For this review, take the finished solid that the model builds, in its own axes (mm). A direction names the side the tool comes from. Give positions to 0.01 mm unless a question says otherwise; leave off trailing zeros. Loops run counter-clockwise (first coordinate to the right, second up) from the corner with the lowest first, then second, coordinate; pieces in that order, holes last. Notation, with made-up numbers: (51.25, 9.25) - (73.25, 9.25) arc R15 ccw to (73.25, 37.25) - close; hole circle Ø11 at (48.25, 88). An arc over 180 degrees is marked (long way). Put each result on its own line as item: value. Start each with the question number.
from build123d import *

# Parameters (mm, degrees)
SKICA1_W                 = 55.6
SKICA1_H                 = 55.6
SKICA1_W_2               = 53.6
SKICA1_H_2               = 53.6
P_IDAT_VYSUNUT_M1_DEPTH  = 10
SKICA3_W                 = 5.8
SKICA3_H                 = 5.8
P_IDAT_VYSUNUT_M2_DEPTH  = 10
ZAOBLIT1_R               = 2.5
SKICA4_R                 = 2.4
ODEBRAT_VYSUNUT_M1_DEPTH = 8
SKICA5_R                 = 0.5
ODEBRAT_VYSUNUT_M2_DEPTH = 2
SKICA6_W                 = 48.6
SKICA6_H                 = 48
ODEBRAT_VYSUNUT_M3_DEPTH = 1.5
SKICA7_W                 = 5.5
SKICA7_H                 = 10.4
ODEBRAT_VYSUNUT_M4_DEPTH = 55.6


with BuildPart() as part:
    # Skica1 → Přidat vysunutím1 (new body)
    with BuildSketch(Plane.XY):
        Rectangle(SKICA1_W, SKICA1_H)
        Rectangle(SKICA1_W_2, SKICA1_H_2, mode=Mode.SUBTRACT)
    extrude(amount=P_IDAT_VYSUNUT_M1_DEPTH)

    # Skica3 → Přidat vysunutím2 (add)
    with BuildSketch(Plane(origin=(0, 0, 0), x_dir=(-1, 0, 0), z_dir=(0, 0, -1))):
        with Locations((23.9, -23.9)):
            Rectangle(SKICA3_W, SKICA3_H)
        with Locations((23.9, 23.9)):
            Rectangle(SKICA3_W, SKICA3_H)
        with Locations((-23.9, -23.9)):
            Rectangle(SKICA3_W, SKICA3_H)
        with Locations((-23.9, 23.9)):
            Rectangle(SKICA3_W, SKICA3_H)
    extrude(amount=-P_IDAT_VYSUNUT_M2_DEPTH)

    # Zaoblit1
    zaoblit1_edges = [part.edges().sort_by_distance(p)[0] for p in [
        (-21, 21, 5),
        (-21, -21, 5),
        (21, -21, 5),
        (21, 21, 5),
    ]]
    fillet(zaoblit1_edges, radius=ZAOBLIT1_R)

    # Skica4 → Odebrat vysunutím1 (cut)
    with BuildSketch(Plane(origin=(0, 0, 0), x_dir=(-1, 0, 0), z_dir=(0, 0, -1))):
        with Locations((23.9, 23.9)):
            Circle(SKICA4_R)
        with Locations((23.9, -23.9)):
            Circle(SKICA4_R)
        with Locations((-23.9, -23.9)):
            Circle(SKICA4_R)
        with Locations((-23.9, 23.9)):
            Circle(SKICA4_R)
    extrude(amount=-ODEBRAT_VYSUNUT_M1_DEPTH, mode=Mode.SUBTRACT)

    # Skica5 → Odebrat vysunutím2 (cut)
    with BuildSketch(Plane(origin=(0, 0, 8), x_dir=(-1, 0, 0), z_dir=(0, 0, -1))):
        with Locations((24.868963017, 24.910500208)):
            Circle(SKICA5_R)
        with Locations((-24.910500208, 24.868963017)):
            Circle(SKICA5_R)
        with Locations((24.910500208, -24.868963017)):
            Circle(SKICA5_R)
        with Locations((-24.868963017, -24.910500208)):
            Circle(SKICA5_R)
    extrude(amount=-ODEBRAT_VYSUNUT_M2_DEPTH, mode=Mode.SUBTRACT)

    # Skica6 → Odebrat vysunutím3 (cut)
    with BuildSketch(Plane.XY.offset(10)):
        Rectangle(SKICA6_W, SKICA6_H)
    extrude(amount=-ODEBRAT_VYSUNUT_M3_DEPTH, mode=Mode.SUBTRACT)

    # Skica7 → Odebrat vysunutím4 (cut)
    with BuildSketch(Plane(origin=(27.8, 0, 0), x_dir=(0, 0, -1), z_dir=(1, 0, 0))):
        with Locations((-4.75, 0)):
            Rectangle(SKICA7_W, SKICA7_H)
    extrude(amount=-ODEBRAT_VYSUNUT_M4_DEPTH, mode=Mode.SUBTRACT)


solid = part.part
1) Take a section at C-C on x = -13.5. State the section outline as (y, z) points.
2) Take a section at A-A on z = 3.25. State how many separate pieces and enclosed holes the cut face has, and give its area (3 significant figures).
3) Mouldability with a two-part tool opening along X and no side actions: class faces 4 (the cylindrical face through (21.713, -21.752, 4.31)), 5 (the flat face through (27.8, -0.4, 1.6)) as released by +X, released by -X, zero draft, split by the parting line, or undercut.
4) Insertion check: P1, Ø1.4, axis at x = 24, y = 24, coming from the -Z side. The pin has a flat end and moves straight along its axis. Give the tip position at first contact, or say it passes through.
5) Machinability: for faces 1 (the flat face through (-23, -22, 8.5)), 2 (the flat face through (21, 25, 5)), 3 (the cylindrical face through (-23.38, 21.557, 3.944)), which of the approach directions +Z, -Z, +X, -X, +Y, -Y give a long, thin tool a straight path to every point of the face, cutting with its end or side? Answer none if there is none.
6) Wall thickness on probe 1 along Y at (x, z) = (-23.9, 3.5); probe 2 along Y at (x, z) = (-16.5, 3); probe 3 along Y at (x, z) = (-22.5, 9.5): over which ranges is each line inside the solid? List them lowest first.
7) Take a section at B-B on y = 2. State the section outline as (x, z) points, and give its area (3 significant figures).
Answers follow:
1. outline: (-27.8, 0) - (-26.8, 0) - (-26.8, 10) - (-27.8, 10) - close; (26.8, 0) - (27.8, 0) - (27.8, 10) - (26.8, 10) - close
2. separate pieces: 2
2. enclosed holes: 4
2. area: 254 mm2
3. face 4: undercut
3. face 5: released by +X
4. P1: z = 8
5. face 1: +Z
5. face 2: +Z, -Z
5. face 3: -Z
6. probe 1: -27.8 to -26.3, -21.5 to -21, 21 to 21.5, 26.3 to 27.8
6. probe 2: -27.8 to -26.8, 26.8 to 27.8
6. probe 3: -27.8 to -24, 24 to 27.8
7. outline: (-27.8, 0) - (-26.8, 0) - (-26.8, 2) - (-27.8, 2) - close; (-27.8, 7.5) - (-26.8, 7.5) - (-26.8, 10) - (-27.8, 10) - close; (26.8, 0) - (27.8, 0) - (27.8, 2) - (26.8, 2) - close; (26.8, 7.5) - (27.8, 7.5) - (27.8, 10) - (26.8, 10) - close
7. area: 9.00 mm2
